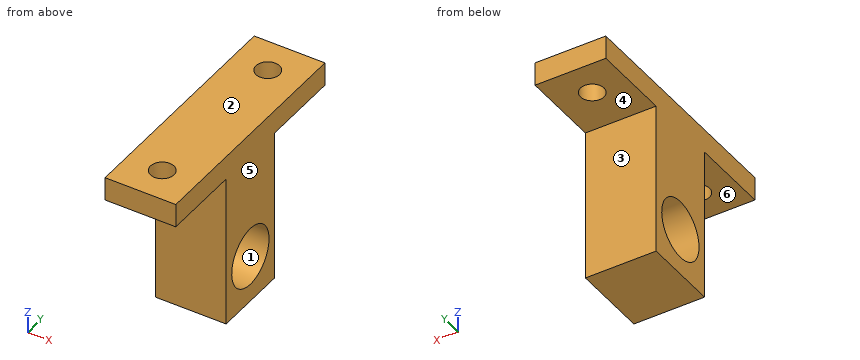
```python
from build123d import *

# Parameters (mm, degrees)
SKETCH1_R           = 5
BOSS_EXTRUDE1_DEPTH = 6
SKETCH2_R           = 2
CUT_EXTRUDE1_DEPTH  = 5


with BuildPart() as part:
    # Sketch1 → Boss-Extrude1 (new body, symmetric)
    with BuildSketch(Plane(origin=(0, 0, 0), x_dir=(0, 0, -1), z_dir=(1, 0, 0))):
        Polygon((-22, -20), (-22, 20), (-18, 20), (-18, 6.5), (8, 6.5), (8, -6.5), (-18, -6.5), (-18, -20), align=None)
        Circle(SKETCH1_R, mode=Mode.SUBTRACT)
    extrude(amount=BOSS_EXTRUDE1_DEPTH, both=True)

    # Sketch2 → Cut-Extrude1 (cut, through all)
    with BuildSketch(Plane(origin=(0, 0, 18), x_dir=(-1, 0, 0), z_dir=(0, 0, -1))):
        with Locations((0, 14.149716829)):
            Circle(SKETCH2_R)
        with Locations((0, -14.149716829)):
            Circle(SKETCH2_R)
    extrude(amount=-CUT_EXTRUDE1_DEPTH, mode=Mode.SUBTRACT)


solid = part.part
```
Geometry check sheet. Reference: the model listing, model coordinates, mm. Face numbers are marked on the shaded views. A direction names the side the tool comes from. Round coordinates to 2 decimals unless told otherwise and drop trailing zeros. Loops run counter-clockwise (first coordinate to the right, second up) from the corner with the lowest first, then second, coordinate; pieces in that order, holes last. Notation, with made-up numbers: (-20, 64) - (7, 64) arc R23 cw to (7, 79) - close; hole circle Ø4 at (-40, -6). An arc over 180 degrees is marked (long way). Write each question's results on one line, items separated by ' | '. Start each with the question number.
Q1. Cross-section at D-D on y = -8. Enter the section's corners in (x, z), and give its area (3 significant figures).
Q2. Release check for a two-part mould opening along Y. For the marked faces 1, 2 and 3 record: +Y half, -Y half, draft (parallel to the pull), parting line (faces both ways), or undercut.
Q3. Access from +Z, -Z, +X, -X, +Y, -Y to the whole of each face (thin tool, end or side, straight path). Record for the marked faces 4, 5 and 6.
Q4. Gauge pin test, flat ends, axial feed: P1, Ø3.5, axis at x = 1.5, z = 11, coming from the -Y side; P2, Ø5, axis at x = 0, y = -14.15, coming from the -Z side; P3, Ø5, axis at x = -2.5, z = 9, coming from the +Y side. Record the tip position at first contact, or that the pin passes through.
Q5. Thickness scan on line 1 (Y direction, x = 0, z = 20.5); line 2 (Z direction, x = -5, y = 13.5); line 3 (Z direction, x = -2.5, y = -3.5). Record the ranges inside material, lowest first. Write a range as [from, to].
Q6. Cross-section at A-A on x = 0. Enter the section's corners in (y, z).
Q7. Cross-section at B-B on y = 0. Enter the section's corners in (x, z).
Q8. Cross-section at C-C on z = 0. Enter the section's corners in (x, y), and give its area (3 significant figures).
Answers below:
1) outline: (-6, 18) - (6, 18) - (6, 22) - (-6, 22) - close | area: 48.0 mm²
2) face 1: undercut | face 2: draft | face 3: +Y half
3) face 4: -Z, +X, -X, +Y | face 5: +Z, -Z, +X, +Y, -Y | face 6: -Z, +X, -X, -Y
4) P1: stops at y = -6.5 | P2: stops at z = 18 | P3: stops at y = 6.5
5) line 1: y = [-20, -16.15], [-12.15, 12.15], [16.15, 20] | line 2: z = [18, 22] | line 3: z = [-8, -3.57], [3.57, 22]
6) outline: (-20, 18) - (-16.15, 18) - (-16.15, 22) - (-20, 22) - close; (-12.15, 18) - (-6.5, 18) - (-6.5, -8) - (6.5, -8) - (6.5, 18) - (12.15, 18) - (12.15, 22) - (-12.15, 22) - close; (16.15, 18) - (20, 18) - (20, 22) - (16.15, 22) - close; hole circle Ø10 at (0, 0)
7) outline: (-6, -8) - (6, -8) - (6, -5) - (-6, -5) - close; (-6, 5) - (6, 5) - (6, 22) - (-6, 22) - close
8) outline: (-6, -6.5) - (6, -6.5) - (6, -5) - (-6, -5) - close; (-6, 5) - (6, 5) - (6, 6.5) - (-6, 6.5) - close | area: 36.0 mm²
